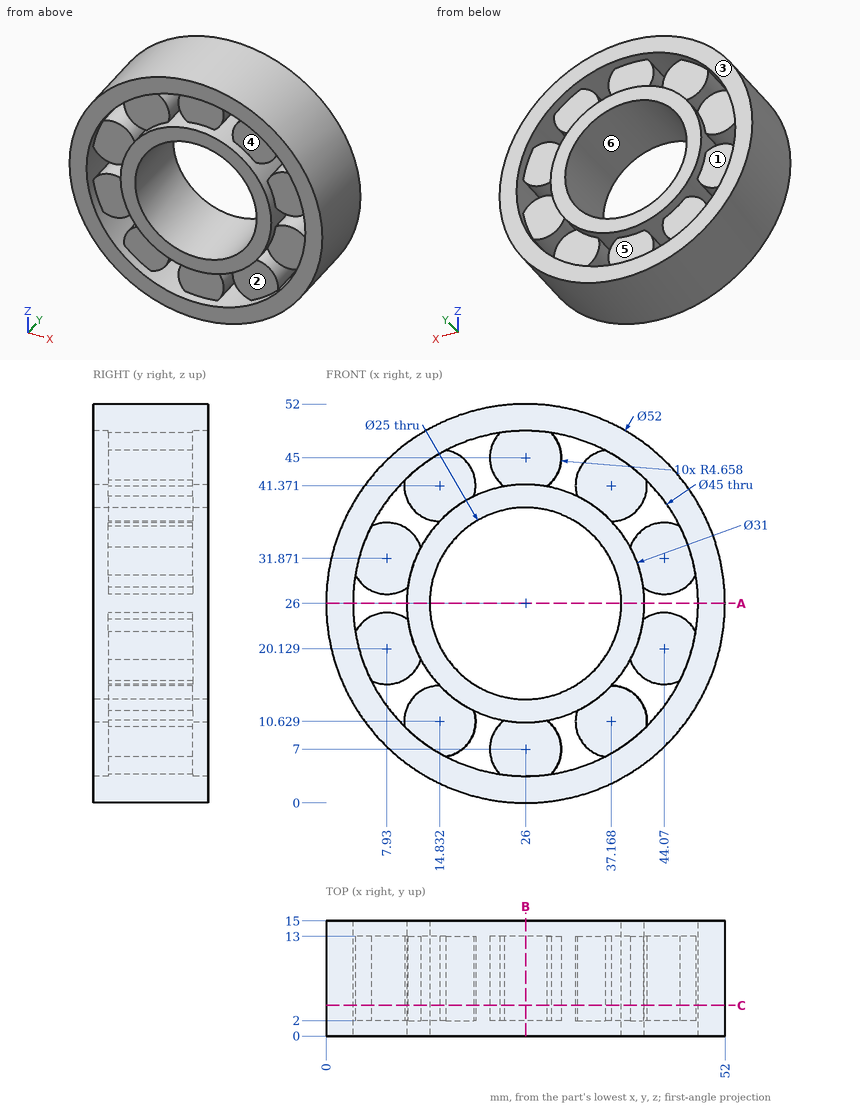
Here's the drawing with two shaded views (mm, measured from the low corner). I have some questions. A direction names the side the tool comes from. Give positions to 0.01 mm unless a question says otherwise; leave off trailing zeros. Write each loop counter-clockwise with the first axis right and the second up, starting at its lowest first coordinate (ties: lowest second). Pieces come first, ordered by that corner, then holes. Notation, with made-up numbers: (13.25, -24.75) -> (71.25, -24.75) arc R25 cw to (71.25, -9.75) -> close; hole circle Ø3 at (-20.75, -8). An arc over 180 degrees is marked (long way). Use one line per item in the form item = value.
1) I'm going to push flat-ended pins straight in: pin 1 (3 mm diameter, centred on x = 21.5, y = 9.5, fed in from +Z); pin 2 (3 mm diameter, centred on x = 14.5, z = 8.5, fed in from -Y); pin 3 (1 mm diameter, centred on y = 10.5, z = 45.5, fed in from -X). Where does each tip first touch, or does it pass through?
Verdict:
pin_1 = 51.83
pin_2 = 2
pin_3 = 8.25
2) Suppose I cut it at C-C (y = 4). Give the number of separate pieces and of enclosed holes in the cut face, and give its area (3 significant figures).
Verdict:
separate_pieces = 1
enclosed_holes = 11
area = 1,380 mm2
3) Suppose I cut it at B-B (x = 26). Please give me the cut outline in (y, z).
Verdict:
outline = (0, 0) -> (15, 0) -> (15, 3.5) -> (13, 3.5) -> (13, 10.5) -> (15, 10.5) -> (15, 13.5) -> (0, 13.5) -> (0, 10.5) -> (2, 10.5) -> (2, 3.5) -> (0, 3.5) -> close; (0, 38.5) -> (15, 38.5) -> (15, 41.5) -> (13, 41.5) -> (13, 48.5) -> (15, 48.5) -> (15, 52) -> (0, 52) -> (0, 48.5) -> (2, 48.5) -> (2, 41.5) -> (0, 41.5) -> close
4) We'd pull the mould along Z, two halves only. Please class the marked faces 1, 2 and 3: +Z half, -Z half, draft (parallel to the pull), parting line (faces both ways), or undercut.
Verdict:
face_1 = undercut
face_2 = undercut
face_3 = draft
5) Suppose I cut it at A-A (z = 26). Please give me the cut outline in (x, y), and give its area (3 significant figures).
Verdict:
outline = (0, 0) -> (3.5, 0) -> (3.5, 15) -> (0, 15) -> close; (10.5, 0) -> (13.5, 0) -> (13.5, 15) -> (10.5, 15) -> close; (38.5, 0) -> (41.5, 0) -> (41.5, 15) -> (38.5, 15) -> close; (48.5, 0) -> (52, 0) -> (52, 15) -> (48.5, 15) -> close
area = 195 mm2
6) If I drill on L1, parallel to Z at x = 26, y = 3.5; L2, parallel to Z at x = 40, y = 5 (1 decimal); L3, parallel to X at y = 10, z = 46.5 (1 decimal), over which ranges is the centre line in solid material (lowest first)? Write a range as [from, to].
Verdict:
L1 = [0, 13.5], [38.5, 52]
L2 = [4.1, 14.3], [17.9, 34.1], [37.7, 47.9]
L3 = [10, 16.7], [21.6, 30.4], [35.3, 42]
7) On a 3-axis mill with a long thin cutter (end or side, diameter ignored), from which of +Z, -Z, +X, -X, +Y, -Y can I reach the whole of each face in a straight line? I mean the marked faces 4, 5 and 6. Say none if no direction works.
Verdict:
face_4 = -Y
face_5 = +Y
face_6 = +Y, -Y
